```python
from build123d import *

# Parameters (mm, degrees)
F1_DEPTH = 10
F2_R     = 4.99999
F3_R     = 2
F4_DEPTH = 25
F5_R     = 4
F6_DEPTH = 3


# Not quite as in the source:
# - a fillet or chamfer is up to 0.001 mm smaller than in the source, because OpenCascade refuses the exact size


with BuildPart() as f1:
    # F0 (on Front) → F1 (new body)
    with BuildSketch(Plane.XZ):
        Polygon((0, 10), (0, 0), (10, 0), (10, 5), (20, 5), (20, 10), align=None)
    extrude(amount=F1_DEPTH)

    # F2 (radius 5 in the source; OpenCascade refuses exactly that, so slightly less here)
    f2_edges = [f1.edges().sort_by_distance(p)[0] for p in [
        (20, -5, 10),
        (0, -5, 10),
    ]]
    fillet(f2_edges, radius=F2_R)

    # F3 (on face) → F4 (cut)
    with BuildSketch(Plane.XY.offset(10)):
        with Locations((5, -5)):
            Circle(F3_R)
    extrude(amount=-F4_DEPTH, mode=Mode.SUBTRACT)

    # F5 (on face) → F6 (cut)
    with BuildSketch(Plane.XY.offset(10)):
        with Locations((5, -5)):
            Circle(F5_R)
    extrude(amount=-F6_DEPTH, mode=Mode.SUBTRACT)


solid = f1.part
```
Geometry check sheet. Reference: the model listing, model coordinates, mm. A direction names the side the tool comes from. Give positions to 0.01 mm unless a question says otherwise; leave off trailing zeros. Order: outer loops, then holes, each group sorted by start corner. A loop starts at its lowest first (then second) coordinate and runs counter-clockwise, first axis right, second up.
1. Access from +Z, -Z, +X, -X, +Y, -Y to the whole of each face (thin tool, end or side, straight path). Record for faces 5 (the face through (15, -5, 5)), 6 (the face through (8, 0, 5)).
2. Section check B-B, the plane z = 4.75. Enter the section's corners in (x, y).
3. Section check D-D, the plane x = 12.25. Enter the section's corners in (y, z), and give its area (3 significant figures).
4. Release check for a two-part mould opening along Y. For faces 1 (the face through (6, -3, 7)), 2 (the face through (8, -10, 5)), 3 (the face through (10, -5, 2)), 4 (the face through (8.695, -6.532, 8.521)) record: pulls with the +Y half, pulls with the -Y half, needs draft (parallel to the pull), parting line crosses it, or undercut.
5. Gauge pin test, flat ends, axial feed: pin 1 Ø4 at (x, y) = (3.5, -5.5) entering from +Z; pin 2 Ø1 at (y, z) = (-2.5, 3.5) entering from +X; pin 3 Ø1 at (x, y) = (11.5, -8.5) entering from -Z. Record the tip position at first contact, or that the pin passes through.
6. Section check C-C, the plane x = 4.5. Enter the section's corners in (y, z).
7. Thickness scan on L1, parallel to Y at x = 5, z = 9.4; L2, parallel to Y at x = 5, z = 6.5; L3, parallel to Z at x = 10.25, y = -7. Record the ranges inside material, lowest first.
Values follow:
1. face 5: -Z, +X, +Y, -Y
1. face 6: +Z, -Z, +X, -X, +Y
2. outline: (0, -10) - (10, -10) - (10, 0) - (0, 0) - close; hole circle Ø4 at (5, -5)
3. outline: (-10, 5) - (0, 5) - (0, 10) - (-10, 10) - close
3. area: 50.0 mm2
4. face 1: undercut
4. face 2: pulls with the -Y half
4. face 3: needs draft
4. face 4: undercut
5. pin 1: stops at z = 7
5. pin 2: stops at x = 10
5. pin 3: stops at z = 5
6. outline: (-10, 0) - (-6.94, 0) - (-6.94, 7) - (-8.97, 7) - (-8.97, 9.97) - (-10, 9.97) - close; (-3.06, 0) - (0, 0) - (0, 9.97) - (-1.03, 9.97) - (-1.03, 7) - (-3.06, 7) - close
7. L1: y = -10 to -9, -1 to 0
7. L2: y = -10 to -7, -3 to 0
7. L3: z = 5 to 10
